Geometry: final body of the model. Coordinates: model frame, mm. Face numbers are marked on the shaded views. A direction names the side the tool comes from. Give positions to 0.01 mm unless a question says otherwise; leave off trailing zeros. Write each loop counter-clockwise with the first axis right and the second up, starting at its lowest first coordinate (ties: lowest second). Pieces come first, ordered by that corner, then holes. Notation, with made-up numbers: M 74,72 L 84,72 A18 ccw 84,91 Z; hole C 74,68 d9. An arc over 180 degrees is marked long. Use a Markdown table: item, result. Add a question column.
1) Draft query along Y for the marked faces 1, 2, 3 and 4. Return one class per face: +Y half, -Y half, draft (parallel to the pull), parting line (faces both ways), or undercut.
2) Section B-B on x = -22.5. Return the cut outline in (y, z), then the cut area to 3 significant figures.
3) Section A-A on z = -7.7. State how many separate pieces and enclosed holes the cut face has, then the cut area to 3 significant figures.
4) Section C-C on y = 115. Return the cut outline in (x, z), then the cut area to 4 significant figures.
5) Line query: line 1 (Y direction, x = -23.75, z = -11); line 2 (X direction, y = 150, z = 1); line 3 (Y direction, x = -24.5, z = 23). Output: solid intervals per line, ascending.
6) Section D-D on z = -2. Return the cut outline in (x, y), then the cut area to 3 significant figures.
7) Set-up query: the marked faces 5, 6 and 7. Return all of +Z, -Z, +X, -X, +Y, -Y with unobstructed straight access to the full face (end or side cutting, diameter ignored); none if empty.
8) Pin query (flat end, axial travel): pin 1 (11 mm diameter, centred on y = 140, z = -6.5, fed in from +X); pin 2 (1.5 mm diameter, centred on x = -26, y = 113, fed in from -Z). Return the tip coordinate at first contact, or that it passes through.
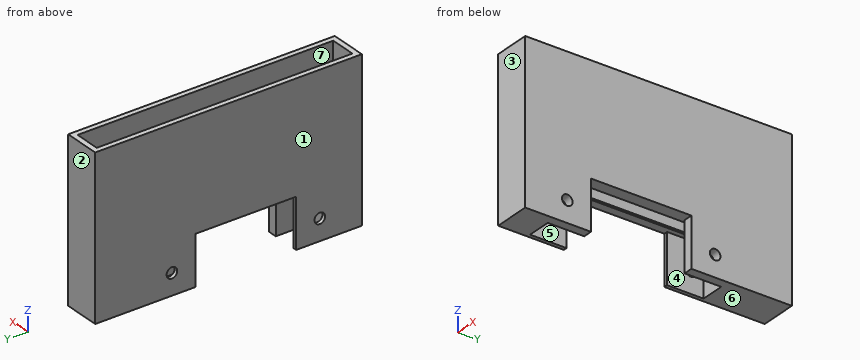
```python
from build123d import *

# Parameters (mm, degrees)
SKETCH_W      = 7.1
SKETCH_H      = 70
SKETCH_W_2    = 4.2
SKETCH_H_2    = 40.5
PAD_DEPTH     = 0.5
SKETCH001_W   = 10
SKETCH001_H   = 73
SKETCH001_W_2 = 7.1
SKETCH001_H_2 = 70
PAD001_DEPTH  = 30
PAD002_DEPTH  = 13.5
SKETCH003_R   = 1.45
HOLE_DEPTH    = 10.001


with BuildPart() as part:
    # Sketch → Pad (new body)
    with BuildSketch(Plane.XY):
        with Locations((-23.097803, 124.895146)):
            Rectangle(SKETCH_W, SKETCH_H)
        with Locations((-23.547803, 120.145146)):
            Rectangle(SKETCH_W_2, SKETCH_H_2, mode=Mode.SUBTRACT)
    extrude(amount=PAD_DEPTH)

    # Sketch001 (on Face9 of Pad) → Pad001 (join)
    with BuildSketch(Plane(origin=(0, 0, 0), x_dir=(1, 0, 0), z_dir=(0, 0, -1))):
        with Locations((-23.097803, -124.895146)):
            Rectangle(SKETCH001_W, SKETCH001_H)
        with Locations((-23.097803, -124.895146)):
            Rectangle(SKETCH001_W_2, SKETCH001_H_2, mode=Mode.SUBTRACT)
    extrude(amount=-PAD001_DEPTH)

    # Sketch002 (on Face15 of Pad001) → Pad002 (join)
    with BuildSketch(Plane(origin=(0, 0, 0), x_dir=(1, 0, 0), z_dir=(0, 0, -1))):
        Polygon((-28.097803, -88.395146), (-28.097803, -96.395146), (-28.097803, -106.395146), (-27.097803, -106.395146), (-27.097803, -96.395146), (-20.597803, -96.395146), (-20.597803, -106.395146), (-18.097803, -106.395146), (-18.097803, -88.395146), align=None)
        Polygon((-28.097803, -161.395146), (-18.097803, -161.395146), (-18.097803, -133.895146), (-20.597803, -133.895146), (-20.597803, -143.895146), (-27.097803, -143.895146), (-27.097803, -133.895146), (-28.097803, -133.895146), (-28.097803, -143.895146), align=None)
    extrude(amount=PAD002_DEPTH)

    # Sketch003 (on Face24 of Pad002) → Hole (cut, through all)
    with BuildSketch(Plane(origin=(-28.097803, 0, 0), x_dir=(0, -1, 0), z_dir=(-1, 0, 0))):
        with Locations((-140.395146, -7.7)):
            Circle(SKETCH003_R)
        with Locations((-99.895146, -7.7)):
            Circle(SKETCH003_R)
    extrude(amount=-HOLE_DEPTH, mode=Mode.SUBTRACT)


solid = part.part
```
Found:
| question | item | result |
|---|---|---|
| 1 | face 1 | draft |
| 1 | face 2 | +Y half |
| 1 | face 3 | -Y half |
| 1 | face 4 | undercut |
| 2 | outline | M 88.4,-13.5 L 96.4,-13.5 L 96.4,0 L 99.9,0 L 99.9,0.5 L 89.9,0.5 L 89.9,30 L 88.4,30 Z; M 140.4,0 L 143.9,0 L 143.9,-13.5 L 161.4,-13.5 L 161.4,30 L 159.9,30 L 159.9,0.5 L 140.4,0.5 Z |
| 2 | area | 449 mm² |
| 3 | separate pieces | 6 |
| 3 | enclosed holes | 0 |
| 3 | area | 305 mm² |
| 4 | outline | M -28.1,0 L -25.65,0 L -25.65,0.5 L -26.65,0.5 L -26.65,30 L -28.1,30 Z; M -21.45,0 L -18.1,0 L -18.1,30 L -19.55,30 L -19.55,0.5 L -21.45,0.5 Z |
| 4 | area | 88.45 mm² |
| 5 | line 1 | 88.4 to 96.4, 143.9 to 161.4 |
| 5 | line 2 | -28.1 to -26.65, -19.55 to -18.1 |
| 5 | line 3 | 88.4 to 89.9, 159.9 to 161.4 |
| 6 | outline | M -28.1,88.4 L -18.1,88.4 L -18.1,106.4 L -20.6,106.4 L -20.6,96.4 L -27.1,96.4 L -27.1,106.4 L -28.1,106.4 Z; M -28.1,133.9 L -27.1,133.9 L -27.1,143.9 L -20.6,143.9 L -20.6,133.9 L -18.1,133.9 L -18.1,161.4 L -28.1,161.4 Z |
| 6 | area | 325 mm² |
| 7 | face 5 | -Z |
| 7 | face 6 | -Z, +X, -X, +Y, -Y |
| 7 | face 7 | +Z |
| 8 | pin 1 | x = -18.1 |
| 8 | pin 2 | z = 0 |
